Design review of the part shown in the three views and the two pictorial views. Dimensions are in mm from the part's minimum x, y and z. Coordinates: 2 decimals unless noted, no trailing zeros. Loops run counter-clockwise (first coordinate to the right, second up) from the corner with the lowest first, then second, coordinate; pieces in that order, holes last. Notation, with made-up numbers: (10.5, 15.25) -> (61.5, 15.25) arc R17 ccw to (61.5, 36.25) -> close; hole circle Ø9 at (54, 80). An arc over 180 degrees is marked (long way). Use a Markdown table: item, result. Add a question column.
Q1. Clearance check with flat-ended pins moving along their axes: pin 1 Ø12 at (y, z) = (15, 39) entering from -X; pin 2 Ø5 at (x, y) = (45.5, 21.5) entering from +Z; pin 3 Ø24.5 at (x, z) = (45, 23) entering from +Y; pin 4 Ø4 at (y, z) = (16.5, 40.5) entering from +X (1 decimal). State where each tip first meets the part, or that it passes through.
Q2. Draft analysis for pull direction X (two halves, no side actions). For the marked faces 1, 2 and 3, state which applies: pulls with the +X half, pulls with the -X half, needs draft (parallel to the pull), parting line crosses it, or undercut.
Q3. Take a section at C-C on x = 22. Write out the cut boundary in (y, z) (1 decimal).
Q4. Take a section at B-B on z = 44. Write out the cut boundary in (x, y) (1 decimal), plus the area to 3 significant figures.
Q5. For probe 1 along Y at (x, z) = (85.5, 21) (1 decimal); probe 2 along Y at (x, z) = (50, 4) (1 decimal); probe 3 along X at (y, z) = (5.5, 13.5) (1 decimal), list the stretches that pass through material, from the lowest coordinate up.
Q6. Take a section at A-A on x = 50. Write out the cut boundary in (y, z) (1 decimal), plus the area to 3 significant figures.
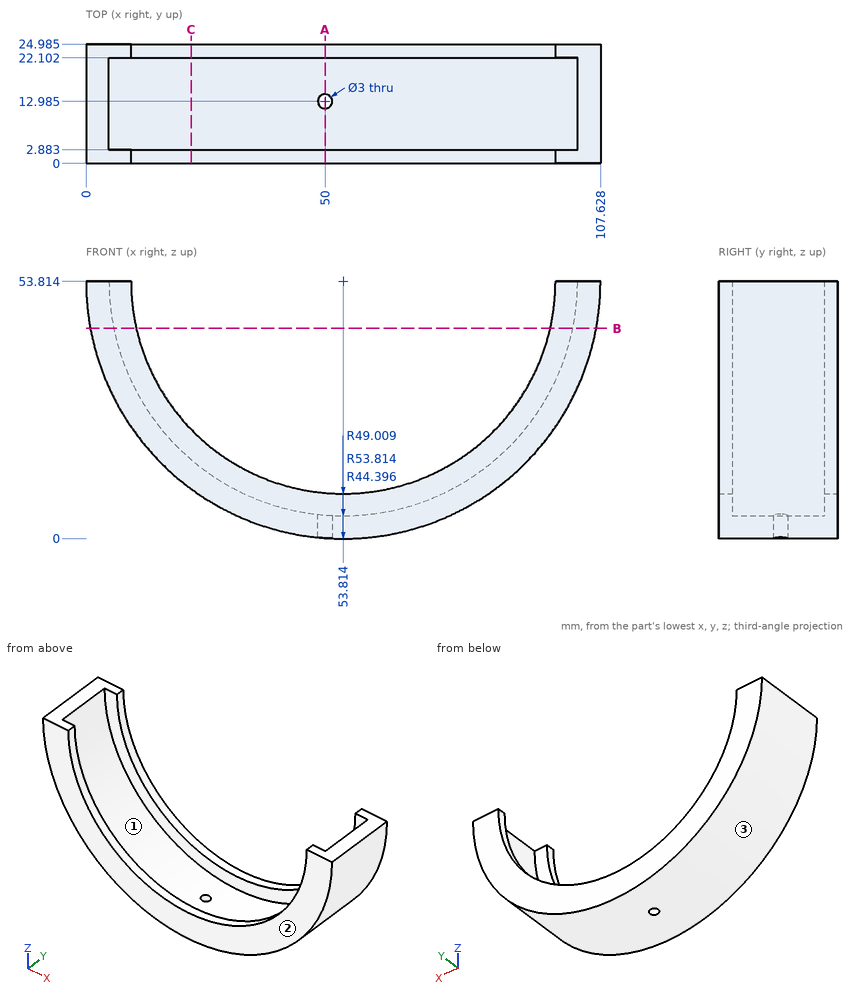
Answer list:
| question | item | result |
|---|---|---|
| 1 | pin 1 | x = 0.73 |
| 1 | pin 2 | z = 10.74 |
| 1 | pin 3 | through |
| 1 | pin 4 | x = 106.4 |
| 2 | face 1 | undercut |
| 2 | face 2 | needs draft |
| 2 | face 3 | parting line crosses it |
| 3 | outline | (0, 10.4) -> (25, 10.4) -> (25, 22.8) -> (22.1, 22.8) -> (22.1, 16.5) -> (2.9, 16.5) -> (2.9, 22.8) -> (0, 22.8) -> close |
| 4 | outline | (0.9, 0) -> (10.5, 0) -> (10.5, 2.9) -> (5.8, 2.9) -> (5.8, 22.1) -> (10.5, 22.1) -> (10.5, 25) -> (0.9, 25) -> close; (97.1, 0) -> (106.7, 0) -> (106.7, 25) -> (97.1, 25) -> (97.1, 22.1) -> (101.8, 22.1) -> (101.8, 2.9) -> (97.1, 2.9) -> close |
| 4 | area | 299 mm² |
| 5 | probe 1 | 0 to 2.9, 22.1 to 25 |
| 5 | probe 2 | 0 to 11.5, 14.5 to 25 |
| 5 | probe 3 | 18.2 to 25.9, 81.7 to 89.5 |
| 6 | outline | (0, 0.1) -> (11.5, 0.1) -> (11.5, 5) -> (2.9, 5) -> (2.9, 9.6) -> (0, 9.6) -> close; (14.5, 0.1) -> (25, 0.1) -> (25, 9.6) -> (22.1, 9.6) -> (22.1, 5) -> (14.5, 5) -> close |
| 6 | area | 133 mm² |
